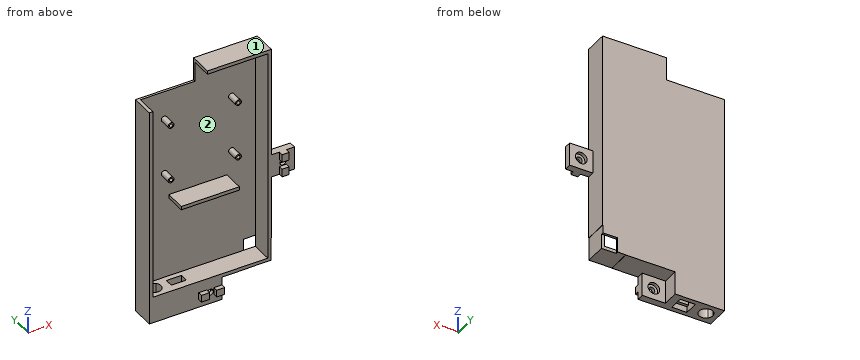
```python
from build123d import *

# Parameters (mm, degrees)
SKETCH_1_W           = 105
SKETCH_1_H           = 170
EXTRUDE_1_DEPTH      = 2
SKETCH_2_W           = 23
SKETCH_2_H           = 20
EXTRUDE_2_DEPTH      = 20
SKETCH_3_W           = 20
SKETCH_3_H           = 20
CUT_EXTRUDE_1_DEPTH  = 14
CUT_EXTRUDE_2_DEPTH  = 14
SKETCH_5_R           = 5
SKETCH_5_R_2         = 2.6
CUT_EXTRUDE_3_DEPTH  = 3
SKETCH_6_W           = 3
SKETCH_6_H           = 75
EXTRUDE_3_DEPTH      = 18
SKETCH_7_W           = 102
SKETCH_7_H           = 3
EXTRUDE_4_DEPTH      = 18
SKETCH_8_W           = 20
SKETCH_8_H           = 20
EXTRUDE_5_DEPTH      = 6
CUT_EXTRUDE_4_DEPTH  = 6
SKETCH_10_R          = 5
SKETCH_10_R_2        = 2.6
CUT_EXTRUDE_5_DEPTH  = 3
SKETCH_11_W          = 6.1
SKETCH_11_H          = 6.95
EXTRUDE_6_DEPTH      = 4
SKETCH_12_W          = 6.95
SKETCH_12_H          = 6.1
EXTRUDE_7_DEPTH      = 4
SKETCH_13_W          = 55
SKETCH_13_H          = 3
EXTRUDE_8_DEPTH      = 20
SKETCH_14_W          = 20
SKETCH_14_H          = 20
CUT_EXTRUDE_6_DEPTH  = 2
SKETCH_15_W          = 42.5
SKETCH_15_H          = 20
EXTRUDE_9_DEPTH      = 20
CUT_EXTRUDE_7_DEPTH  = 30
CUT_EXTRUDE_9_DEPTH  = 30
SKETCH_19_W          = 19.8
SKETCH_19_H          = 0.2
CUT_EXTRUDE_10_DEPTH = 30
EXTRUDE_17_DEPTH     = 2
CUT_EXTRUDE_11_DEPTH = 5
SKETCH_25_W          = 52
SKETCH_25_H          = 3
CUT_EXTRUDE_12_DEPTH = 18
SKETCH_26_W          = 105
SKETCH_26_H          = 20
EXTRUDE_18_DEPTH     = 2
SKETCH_27_W          = 52
SKETCH_27_H          = 3
EXTRUDE_19_DEPTH     = 18
SKETCH_28_W          = 50
SKETCH_28_H          = 20
CUT_EXTRUDE_13_DEPTH = 18
SKETCH_29_W          = 3
SKETCH_29_H          = 167
EXTRUDE_20_DEPTH     = 18
SKETCH_30_R          = 2.5
SKETCH_30_R_2        = 1.48
EXTRUDE_21_DEPTH     = 10
SKETCH_31_R          = 1.48
EXTRUDE_22_DEPTH     = 2
EXTRUDE_24_DEPTH     = 18


with BuildPart() as part:
    # Sketch 1 → Extrude 1 (new body)
    with BuildSketch(Plane(origin=(0, 0, 0), x_dir=(1, 0, 0), z_dir=(0, 1, 0))):
        with Locations((52.5, 85)):
            Rectangle(SKETCH_1_W, SKETCH_1_H)
    extrude(amount=EXTRUDE_1_DEPTH)

    # Sketch 2 → Extrude 2 (add)
    with BuildSketch(Plane(origin=(0, 2, 0), x_dir=(1, 0, 0), z_dir=(0, 1, 0))):
        with Locations((113.5, 85)):
            Rectangle(SKETCH_2_W, SKETCH_2_H)
    extrude(amount=-EXTRUDE_2_DEPTH)

    # Sketch 3 → Cut-Extrude 1 (cut)
    with BuildSketch(Plane(origin=(0, 2, 0), x_dir=(1, 0, 0), z_dir=(0, 1, 0))):
        with Locations((115, 85)):
            Rectangle(SKETCH_3_W, SKETCH_3_H)
    extrude(amount=-CUT_EXTRUDE_1_DEPTH, mode=Mode.SUBTRACT)

    # Sketch 4 → Cut-Extrude 2 (cut)
    with BuildSketch(Plane(origin=(0, -12, 0), x_dir=(1, 0, 0), z_dir=(0, 1, 0))):
        with BuildLine():
            ThreePointArc((117.6, 85), (115.994976924, 87.402086785), (113.161522369, 86.838477631))
            Line((113.161522369, 86.838477631), (116.838477631, 83.161522369))
            ThreePointArc((116.838477631, 83.161522369), (117.402086785, 84.005023076), (117.6, 85))
        make_face()
        with BuildLine():
            Line((116.838477631, 83.161522369), (113.161522369, 86.838477631))
            ThreePointArc((113.161522369, 86.838477631), (113.161522369, 83.161522369), (116.838477631, 83.161522369))
        make_face()
    extrude(amount=-CUT_EXTRUDE_2_DEPTH, mode=Mode.SUBTRACT)

    # Sketch 5 → Cut-Extrude 3 (cut)
    with BuildSketch(Plane(origin=(0, -12, 0), x_dir=(1, 0, 0), z_dir=(0, 1, 0))):
        with Locations(Location((115, 85, 0), (0, 0, 270))):
            Circle(SKETCH_5_R)
        with Locations(Location((115, 85, 0), (0, 0, 270))):
            Circle(SKETCH_5_R_2, mode=Mode.SUBTRACT)
    extrude(amount=-CUT_EXTRUDE_3_DEPTH, mode=Mode.SUBTRACT)

    # Sketch 6 → Extrude 3 (add)
    with BuildSketch(Plane.XZ):
        with Locations((103.5, -132.5)):
            Rectangle(SKETCH_6_W, SKETCH_6_H)
        with Locations((103.5, -37.5)):
            Rectangle(SKETCH_6_W, SKETCH_6_H)
    extrude(amount=EXTRUDE_3_DEPTH)

    # Sketch 7 → Extrude 4 (add)
    with BuildSketch(Plane(origin=(0, 0, 0), x_dir=(-1, 0, 0), z_dir=(0, -1, 0))):
        with Locations((-51, 168.5)):
            Rectangle(SKETCH_7_W, SKETCH_7_H)
    extrude(amount=EXTRUDE_4_DEPTH)

    # Sketch 8 → Extrude 5 (add)
    with BuildSketch(Plane(origin=(0, -18, 0), x_dir=(-1, 0, 0), z_dir=(0, -1, 0))):
        with Locations((-52.5, 180)):
            Rectangle(SKETCH_8_W, SKETCH_8_H)
    extrude(amount=-EXTRUDE_5_DEPTH)

    # Sketch 9 → Cut-Extrude 4 (cut)
    with BuildSketch(Plane(origin=(0, -12, 0), x_dir=(1, 0, 0), z_dir=(0, 1, 0))):
        with BuildLine():
            ThreePointArc((55.1, 180), (53.494976924, 182.402086785), (50.661522369, 181.838477631))
            Line((50.661522369, 181.838477631), (54.338477631, 178.161522369))
            ThreePointArc((54.338477631, 178.161522369), (54.902086785, 179.005023076), (55.1, 180))
        make_face()
        with BuildLine():
            Line((54.338477631, 178.161522369), (50.661522369, 181.838477631))
            ThreePointArc((50.661522369, 181.838477631), (50.661522369, 178.161522369), (54.338477631, 178.161522369))
        make_face()
    extrude(amount=-CUT_EXTRUDE_4_DEPTH, mode=Mode.SUBTRACT)

    # Sketch 10 → Cut-Extrude 5 (cut)
    with BuildSketch(Plane(origin=(0, -12, 0), x_dir=(1, 0, 0), z_dir=(0, 1, 0))):
        with Locations(Location((52.5, 180, 0), (0, 0, 270))):
            Circle(SKETCH_10_R)
        with Locations(Location((52.5, 180, 0), (0, 0, 270))):
            Circle(SKETCH_10_R_2, mode=Mode.SUBTRACT)
    extrude(amount=-CUT_EXTRUDE_5_DEPTH, mode=Mode.SUBTRACT)

    # Sketch 11 → Extrude 6 (add)
    with BuildSketch(Plane.XZ.offset(18)):
        Polygon((118.05, -88.05), (115, -88.05), (111.95, -88.05), (111.95, -95), (118.05, -95), align=None)
        with Locations((115, -78.475)):
            Rectangle(SKETCH_11_W, SKETCH_11_H)
    extrude(amount=EXTRUDE_6_DEPTH)

    # Sketch 12 → Extrude 7 (add)
    with BuildSketch(Plane(origin=(0, -18, 0), x_dir=(-1, 0, 0), z_dir=(0, -1, 0))):
        Polygon((-49.45, 183.05), (-49.45, 180), (-49.45, 176.95), (-42.5, 176.95), (-42.5, 183.05), align=None)
        with Locations((-59.025, 180)):
            Rectangle(SKETCH_12_W, SKETCH_12_H)
    extrude(amount=EXTRUDE_7_DEPTH)

    # Sketch 13 → Extrude 8 (add)
    with BuildSketch(Plane(origin=(0, 2, 0), x_dir=(1, 0, 0), z_dir=(0, 1, 0))):
        with Locations((77.5, 1.5)):
            Rectangle(SKETCH_13_W, SKETCH_13_H)
    extrude(amount=-EXTRUDE_8_DEPTH)

    # Sketch 14 → Cut-Extrude 6 (cut)
    with BuildSketch(Plane(origin=(0, 2, 0), x_dir=(1, 0, 0), z_dir=(0, 1, 0))):
        with Locations((95, 160)):
            Rectangle(SKETCH_14_W, SKETCH_14_H)
    extrude(amount=-CUT_EXTRUDE_6_DEPTH, mode=Mode.SUBTRACT)

    # Sketch 15 → Extrude 9 (add)
    with BuildSketch(Plane.XZ.offset(18)):
        with Locations((21.25, -180)):
            Rectangle(SKETCH_15_W, SKETCH_15_H)
    extrude(amount=-EXTRUDE_9_DEPTH)

    # Sketch 16 → Cut-Extrude 7 (cut)
    with BuildSketch(Plane(origin=(0, 0, -190), x_dir=(-1, 0, 0), z_dir=(0, 0, -1))):
        with BuildLine():
            ThreePointArc((-4, -8), (-7.703899406, -2.456722805), (-14.242640687, -3.757359313))
            Line((-14.242640687, -3.757359313), (-5.757359313, -12.242640687))
            ThreePointArc((-5.757359313, -12.242640687), (-4.456722805, -10.296100594), (-4, -8))
        make_face()
        with BuildLine():
            Line((-5.757359313, -12.242640687), (-14.242640687, -3.757359313))
            ThreePointArc((-14.242640687, -3.757359313), (-14.242640687, -12.242640687), (-5.757359313, -12.242640687))
        make_face()
    extrude(amount=-CUT_EXTRUDE_7_DEPTH, mode=Mode.SUBTRACT)

    # Sketch 17 → Cut-Extrude 9 (cut)
    with BuildSketch(Plane(origin=(0, 0, -190), x_dir=(-1, 0, 0), z_dir=(0, 0, -1))):
        Polygon((-22.75, -4.5), (-29.25, -4.5), (-35.75, -4.5), (-35.75, -11.5), (-29.25, -11.5), (-22.75, -11.5), align=None)
    extrude(amount=-CUT_EXTRUDE_9_DEPTH, mode=Mode.SUBTRACT)

    # Sketch 19 → Cut-Extrude 10 (cut)
    with BuildSketch(Plane(origin=(0, 0, 0), x_dir=(1, 0, 0), z_dir=(0, 1, 0))):
        with Locations((94.9, 169.9)):
            Rectangle(SKETCH_19_W, SKETCH_19_H)
        Polygon((105, 150), (105, 170), (104.8, 170), (104.8, 169.8), (104.8, 150), align=None)
    extrude(amount=-CUT_EXTRUDE_10_DEPTH, mode=Mode.SUBTRACT)

    # Sketch 21 → Extrude 17 (add)
    with BuildSketch(Plane(origin=(0, 2, 0), x_dir=(1, 0, 0), z_dir=(0, 1, 0))):
        Polygon((102, 157), (92, 157), (92, 167), (92, 169.8), (85, 169.8), (85, 167), (85, 150), (102, 150), (104.8, 150), (104.8, 157), align=None)
    extrude(amount=-EXTRUDE_17_DEPTH)

    # Sketch 23 → Cut-Extrude 11 (cut)
    with BuildSketch(Plane(origin=(0, 0, -190), x_dir=(-1, 0, 0), z_dir=(0, 0, -1))):
        Polygon((-22.75, -11.5), (-22.75, -14), (-35.75, -14), (-35.75, -2), (-22.75, -2), align=None)
    extrude(amount=-CUT_EXTRUDE_11_DEPTH, mode=Mode.SUBTRACT)

    # Sketch 25 → Cut-Extrude 12 (cut)
    with BuildSketch(Plane(origin=(0, -18, 0), x_dir=(-1, 0, 0), z_dir=(0, -1, 0))):
        with Locations((-76, 1.5)):
            Rectangle(SKETCH_25_W, SKETCH_25_H)
    extrude(amount=-CUT_EXTRUDE_12_DEPTH, mode=Mode.SUBTRACT)

    # Sketch 26 → Extrude 18 (add)
    with BuildSketch(Plane(origin=(0, 2, 0), x_dir=(1, 0, 0), z_dir=(0, 1, 0))):
        with Locations((52.5, -10)):
            Rectangle(SKETCH_26_W, SKETCH_26_H)
    extrude(amount=-EXTRUDE_18_DEPTH)

    # Sketch 27 → Extrude 19 (add)
    with BuildSketch(Plane(origin=(0, 0, 0), x_dir=(-1, 0, 0), z_dir=(0, -1, 0))):
        with Locations((-76, -18.5)):
            Rectangle(SKETCH_27_W, SKETCH_27_H)
        Polygon((-102, -17), (-102, 0), (-105, 0), (-105, -20), (-102, -20), align=None)
    extrude(amount=EXTRUDE_19_DEPTH)

    # Sketch 28 → Cut-Extrude 13 (cut)
    with BuildSketch(Plane.XZ):
        with Locations((25, 10)):
            Rectangle(SKETCH_28_W, SKETCH_28_H)
    extrude(amount=-CUT_EXTRUDE_13_DEPTH, mode=Mode.SUBTRACT)

    # Sketch 29 → Extrude 20 (add)
    with BuildSketch(Plane(origin=(0, 0, 0), x_dir=(-1, 0, 0), z_dir=(0, -1, 0))):
        with Locations((-1.5, 83.5)):
            Rectangle(SKETCH_29_W, SKETCH_29_H)
    extrude(amount=EXTRUDE_20_DEPTH)

    # Sketch 30 → Extrude 21 (add)
    # profile 1 of 4: a face of its own
    with BuildSketch(Plane.XZ):
        with Locations(Location((23.5, -24.5, 0), (0, 0, 90))):
            Circle(SKETCH_30_R)
        with Locations(Location((23.5, -24.5, 0), (0, 0, 270))):
            Circle(SKETCH_30_R_2, mode=Mode.SUBTRACT)
    # profile 2 of 4: a face of its own
    with BuildSketch(Plane.XZ):
        with Locations(Location((81.5, -24.5, 0), (0, 0, 90))):
            Circle(SKETCH_30_R)
        with Locations(Location((81.5, -24.5, 0), (0, 0, 270))):
            Circle(SKETCH_30_R_2, mode=Mode.SUBTRACT)
    # profile 3 of 4: a face of its own
    with BuildSketch(Plane.XZ):
        with Locations(Location((23.5, -73.5, 0), (0, 0, 90))):
            Circle(SKETCH_30_R)
        with Locations(Location((23.5, -73.5, 0), (0, 0, 270))):
            Circle(SKETCH_30_R_2, mode=Mode.SUBTRACT)
    # profile 4 of 4: a face of its own
    with BuildSketch(Plane.XZ):
        with Locations(Location((81.5, -73.5, 0), (0, 0, 90))):
            Circle(SKETCH_30_R)
        with Locations(Location((81.5, -73.5, 0), (0, 0, 270))):
            Circle(SKETCH_30_R_2, mode=Mode.SUBTRACT)
    extrude(amount=EXTRUDE_21_DEPTH)

    # Sketch 31 → Extrude 22 (add)
    with BuildSketch(Plane.XZ):
        with Locations(Location((23.5, -24.5, 0), (0, 0, 270))):
            Circle(SKETCH_31_R)
        with Locations(Location((81.5, -24.5, 0), (0, 0, 270))):
            Circle(SKETCH_31_R)
        with Locations(Location((81.5, -73.5, 0), (0, 0, 270))):
            Circle(SKETCH_31_R)
        with Locations(Location((23.5, -73.5, 0), (0, 0, 270))):
            Circle(SKETCH_31_R)
    extrude(amount=EXTRUDE_22_DEPTH)

    # Sketch 33 → Extrude 24 (add)
    with BuildSketch(Plane.XZ):
        Polygon((77.5, -94), (77.5, -97), (52.5, -97), (27.5, -97), (27.5, -94), align=None)
    extrude(amount=EXTRUDE_24_DEPTH)


solid = part.part
```
Geometry check sheet. Reference: the model listing, model coordinates, mm. Face numbers are marked on the shaded views. A direction names the side the tool comes from. Round coordinates to 2 decimals unless told otherwise and drop trailing zeros. Order: outer loops, then holes, each group sorted by start corner. A loop starts at its lowest first (then second) coordinate and runs counter-clockwise, first axis right, second up. Notation, with made-up numbers: (67, 10.5) - (101, 10.5) arc R32 cw to (101, 46.5) - close; hole circle Ø9 at (5, -38.5). An arc over 180 degrees is marked (long way). Use a Markdown table: item, result. Add a question column.
1) Section check C-C (x = 69.5). Record the cut outline in (y, z).
2) Gauge pin test, flat ends, axial feed: P1, Ø10, axis at y = -5, z = -54.5, coming from the +X side; P2, Ø4.5, axis at y = -19, z = -181, coming from the -X side; P3, Ø3, axis at y = -20.5, z = -181, coming from the -X side; P4, Ø4, axis at x = 81.5, z = -25.5, coming from the -Y side. Record the tip position at first contact, or that the pin passes through.
3) Section check A-A (x = 10). Record the cut outline in (y, z), then the cut area to 3 significant figures.
4) Section check B-B (z = -159.5). Record the cut outline in (x, y).
5) Set-up check for the marked faces 1 and 2: record each of +Z, -Z, +X, -X, +Y, -Y from which the full face is reachable in a straight line by a thin tool's end or side.
6) Section check D-D (x = 90). Record the cut outline in (y, z).
7) Thickness scan on line 1 along X through (y, z) = (-4.75, -73.5); line 2 along X through (y, z) = (-14.75, -96); line 3 along Z through (x, y) = (63, -13.75). Record the ranges inside material, lowest first.
Established:
| question | item | result |
|---|---|---|
| 1 | outline | (-18, -170) - (2, -170) - (2, 20) - (-18, 20) - (-18, 17) - (0, 17) - (0, -94) - (-18, -94) - (-18, -97) - (0, -97) - (0, -167) - (-18, -167) - close |
| 2 | P1 | x = 105 |
| 2 | P2 | x = 0 |
| 2 | P3 | x = 42.5 |
| 2 | P4 | y = -10 |
| 3 | outline | (-18, -190) - (-14, -190) - (-14, -167) - (-18, -167) - close; (-2, -190) - (2, -190) - (2, 0) - (0, 0) - (0, -167) - (-2, -167) - close |
| 3 | area | 518 mm2 |
| 4 | outline | (0, -18) - (3, -18) - (3, 0) - (92, 0) - (92, 2) - (0, 2) - close; (102, -18) - (104.8, -18) - (104.8, 0) - (102, 0) - close |
| 5 | face 1 | +Z, +X, -X, +Y, -Y |
| 5 | face 2 | -Y |
| 6 | outline | (-18, -169.8) - (2, -169.8) - (2, 20) - (-18, 20) - (-18, 17) - (0, 17) - (0, -167) - (-18, -167) - close |
| 7 | line 1 | 0 to 3, 21 to 22.02, 24.98 to 26, 79 to 80.02, 82.98 to 84, 102 to 105 |
| 7 | line 2 | 0 to 3, 27.5 to 77.5, 102 to 105 |
| 7 | line 3 | -170 to -167, -97 to -94, 17 to 20 |
